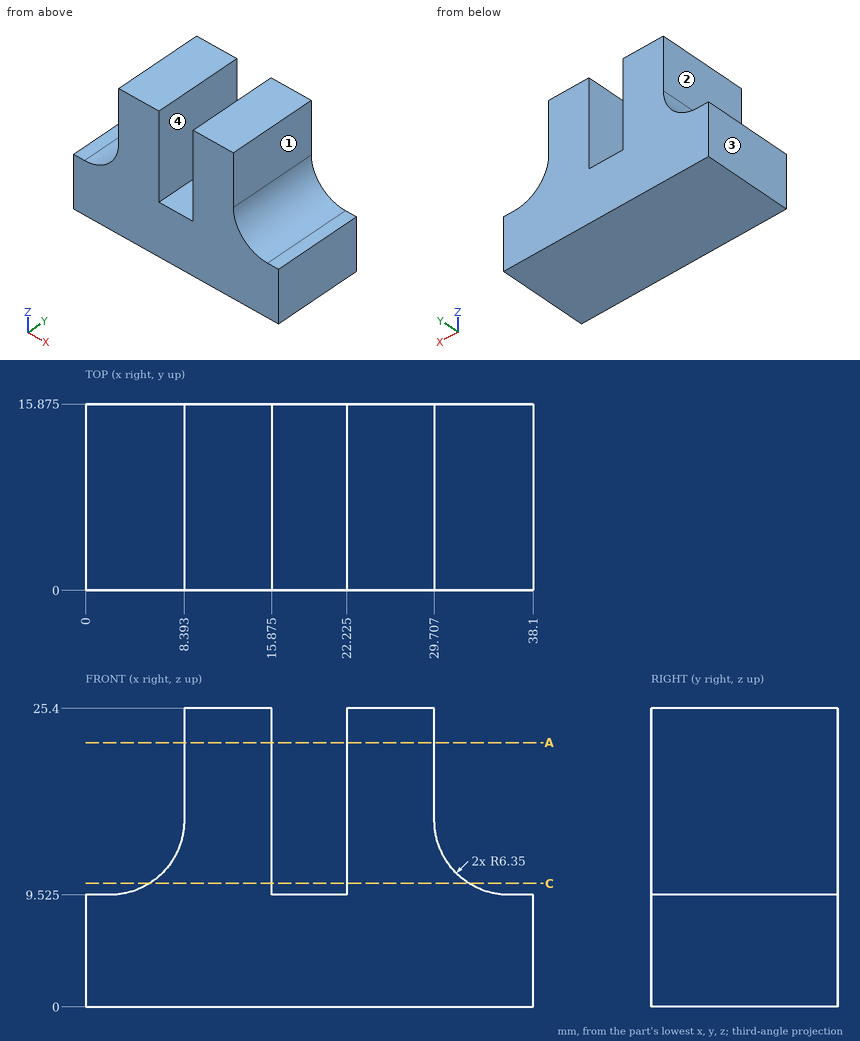
Source: three-view drawing plus pictorial views. Frame: mm from the lowest corner of the part. A direction names the side the tool comes from. Round coordinates to 2 decimals unless told otherwise and drop trailing zeros. Order: outer loops, then holes, each group sorted by start corner. A loop starts at its lowest first (then second) coordinate and runs counter-clockwise, first axis right, second up. Notation, with made-up numbers: M 12.5,56.5 L 32.5,56.5 A12 ccw 32.5,68.5 Z; hole C 86.5,22.5 d9. An arc over 180 degrees is marked long. One line per item, written item: value.
(1) Cut plane C-C (z = 10.5). Return the cut outline in (x, y) (1 decimal), and give its area (3 significant figures).
Result sheet:
outline: M 5.4,0 L 15.9,0 L 15.9,15.9 L 5.4,15.9 Z; M 22.2,0 L 32.7,0 L 32.7,15.9 L 22.2,15.9 Z
area: 332 mm2
(2) Cut plane A-A (z = 22.5). Return the cut outline in (x, y) (1 decimal).
Result sheet:
outline: M 8.4,0 L 15.9,0 L 15.9,15.9 L 8.4,15.9 Z; M 22.2,0 L 29.7,0 L 29.7,15.9 L 22.2,15.9 Z
(3) Line query: probe 1 along X at (y, z) = (1.5, 22.75) (1 decimal); probe 2 along X at (y, z) = (2.5, 12.5) (1 decimal); probe 3 along Z at (x, y) = (36, 10) (1 decimal). Output: solid intervals per line, ascending. Write a range as [from, to].
Result sheet:
probe 1: [8.4, 15.9], [22.2, 29.7]
probe 2: [7.4, 15.9], [22.2, 30.7]
probe 3: [0, 9.5]
(4) Reachability of the marked faces 1, 2, 3 and 4 from +Z, -Z, +X, -X, +Y, -Y: full face, straight path, thin tool, end or side. Return the list, or none.
Result sheet:
face 1: +Z, +X, +Y, -Y
face 2: +Z, -X, +Y, -Y
face 3: +Z, -Z, -X, +Y, -Y
face 4: +Z, +Y, -Y
(5) Pin query (flat end, axial travel): P1, Ø1.9, axis at x = 20.5, y = 6, coming from the +Z side (3 decimals); P2, Ø5, axis at y = 7.5, z = 16.5, coming from the -X side; P3, Ø7.5, axis at y = 6, z = 21, coming from the -X side. Return the tip coordinate at first contact, or that it passes through.
Result sheet:
P1: z = 9.525
P2: x = 8.11
P3: x = 8.39
